```python
from build123d import *

# Parameters (mm, degrees)
SKETCH1_W                        = 279.4
SKETCH1_H                        = 76.2
BOSS_EXTRUDE1_DEPTH              = 6.35
F_25_32_0_78125_DIAMETER_HOLE1_D = 19.84375
SKETCH6_R                        = 3.302
CUT_EXTRUDE1_DEPTH               = 6.35
CIRPATTERN1_COUNT                = 4
MIRROR2_COPY_1_SKETCH_R          = 3.302
MIRROR2_COPY_1_DEPTH             = 6.35
MIRROR2_COPY_2_SKETCH_R          = 3.302
MIRROR2_COPY_2_DEPTH             = 6.35
MIRROR2_COPY_3_SKETCH_R          = 3.302
MIRROR2_COPY_3_DEPTH             = 6.35
SKETCH7_R                        = 3.556
CUT_EXTRUDE2_DEPTH               = 6.35


with BuildPart() as part:
    # Sketch1 → Boss-Extrude1 (new body)
    with BuildSketch(Plane(origin=(0, 0, 0), x_dir=(1, 0, 0), z_dir=(0, 1, 0))):
        Rectangle(SKETCH1_W, SKETCH1_H)
    extrude(amount=BOSS_EXTRUDE1_DEPTH)

    # 25/32 (0.78125) Diameter Hole1 (through all)
    with Locations(Plane(origin=(0, 6.35, 0), x_dir=(1, 0, 0), z_dir=(0, 1, 0))):
        with Locations((87.3125, 0)):
            f_25_32_0_78125_diameter_hole1 = Hole(F_25_32_0_78125_DIAMETER_HOLE1_D / 2)

    # Sketch6 → Cut-Extrude1 (cut)
    with BuildSketch(Plane(origin=(0, 6.35, 0), x_dir=(1, 0, 0), z_dir=(0, 1, 0))):
        with Locations(Location((60.6425, 0, 0), (0, 0, 270))):
            Circle(SKETCH6_R)
    cut_extrude1 = extrude(amount=-CUT_EXTRUDE1_DEPTH, mode=Mode.SUBTRACT)

    # CirPattern1: Cut-Extrude1 ×4 about axis
    cirpattern1_axis = Axis((87.3125, 0, 0), (0, 1, 0))
    for i in range(1, CIRPATTERN1_COUNT):
        add(cut_extrude1.rotate(cirpattern1_axis, i * 360 / CIRPATTERN1_COUNT), mode=Mode.SUBTRACT)

    # Mirror2: 25/32 (0.78125) Diameter Hole1, Cut-Extrude1 across plane
    add(f_25_32_0_78125_diameter_hole1.mirror(Plane(origin=(0, 0, 0), x_dir=(0, 0, 1), z_dir=(1, 0, 0))), mode=Mode.SUBTRACT)
    add(cut_extrude1.mirror(Plane(origin=(0, 0, 0), x_dir=(0, 0, 1), z_dir=(1, 0, 0))), mode=Mode.SUBTRACT)

    # Mirror2 copy 1 sketch → Mirror2 copy 1 (cut)
    with BuildSketch(Plane(origin=(-87.3125, 6.35, 87.3125), x_dir=(0, 0, -1), z_dir=(0, 1, 0))):
        with Locations((60.6425, 0)):
            Circle(MIRROR2_COPY_1_SKETCH_R)
    extrude(amount=-MIRROR2_COPY_1_DEPTH, mode=Mode.SUBTRACT)

    # Mirror2 copy 2 sketch → Mirror2 copy 2 (cut)
    with BuildSketch(Plane(origin=(-174.625, 6.35, 0), x_dir=(1, 0, 0), z_dir=(0, 1, 0))):
        with Locations((60.6425, 0)):
            Circle(MIRROR2_COPY_2_SKETCH_R)
    extrude(amount=-MIRROR2_COPY_2_DEPTH, mode=Mode.SUBTRACT)

    # Mirror2 copy 3 sketch → Mirror2 copy 3 (cut)
    with BuildSketch(Plane(origin=(-87.3125, 6.35, -87.3125), x_dir=(0, 0, 1), z_dir=(0, 1, 0))):
        with Locations((60.6425, 0)):
            Circle(MIRROR2_COPY_3_SKETCH_R)
    extrude(amount=-MIRROR2_COPY_3_DEPTH, mode=Mode.SUBTRACT)

    # Sketch7 → Cut-Extrude2 (cut)
    with BuildSketch(Plane(origin=(0, 0, 0), x_dir=(-1, 0, 0), z_dir=(0, -1, 0))):
        with Locations(Location((0, 0, 0), (0, 0, 90))):
            Circle(SKETCH7_R)
    extrude(amount=-CUT_EXTRUDE2_DEPTH, mode=Mode.SUBTRACT)


solid = part.part
```
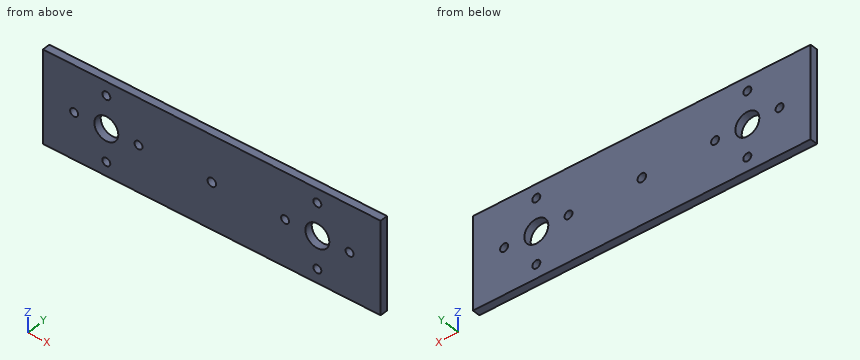
The model under review builds one solid part; all positions refer to its coordinate system, in mm. Round coordinates to 2 decimals unless told otherwise and drop trailing zeros. Loops run counter-clockwise (first coordinate to the right, second up) from the corner with the lowest first, then second, coordinate; pieces in that order, holes last. Notation, with made-up numbers: (2, -23.75) - (38, -23.75) arc R12 ccw to (38, -8.75) - close; hole circle Ø6 at (10, 84). An arc over 180 degrees is marked (long way). Write each question's results on one line, items separated by ' | '. Start each with the question number.
Q1. Take a section at C-C on z = 26.67. Give the boundary of the cut face in (x, y), plus the area to 3 significant figures.
Q2. Take a section at B-B on x = 0. Give the boundary of the cut face in (y, z).
Q3. Insertion check: P1, Ø8.5, axis at x = -113.98, z = 0, coming from the -Y side. The pin has a flat end and moves straight along its axis. Give the tip position at first contact, or say it passes through.
Q4. Wall thickness on line 1 along X through (y, z) = (2.5, 26.67); line 2 along X through (y, z) = (3, -7); line 3 along Z through (x, y) = (-85.5, 0.5): over which ranges is each line inside the solid? List them lowest first. Write a range as [from, to].
Q5. Take a section at A-A on z = 0. Give the number of separate pieces and of enclosed holes in the cut face, plus the area to 3 significant figures.
Data:
1) outline: (-139.7, 0) - (-90.61, 0) - (-90.61, 6.35) - (-139.7, 6.35) - close; (-84.01, 0) - (84.01, 0) - (84.01, 6.35) - (-84.01, 6.35) - close; (90.61, 0) - (139.7, 0) - (139.7, 6.35) - (90.61, 6.35) - close | area: 1,690 mm²
2) outline: (0, -38.1) - (6.35, -38.1) - (6.35, -3.56) - (0, -3.56) - close; (0, 3.56) - (6.35, 3.56) - (6.35, 38.1) - (0, 38.1) - close
3) P1: stops at y = 0
4) line 1: x = [-139.7, -90.61], [-84.01, 84.01], [90.61, 139.7] | line 2: x = [-139.7, -94.34], [-80.28, 80.28], [94.34, 139.7] | line 3: z = [-38.1, -29.43], [-23.91, -9.75], [9.75, 23.91], [29.43, 38.1]
5) separate pieces: 8 | enclosed holes: 0 | area: 1,310 mm²
